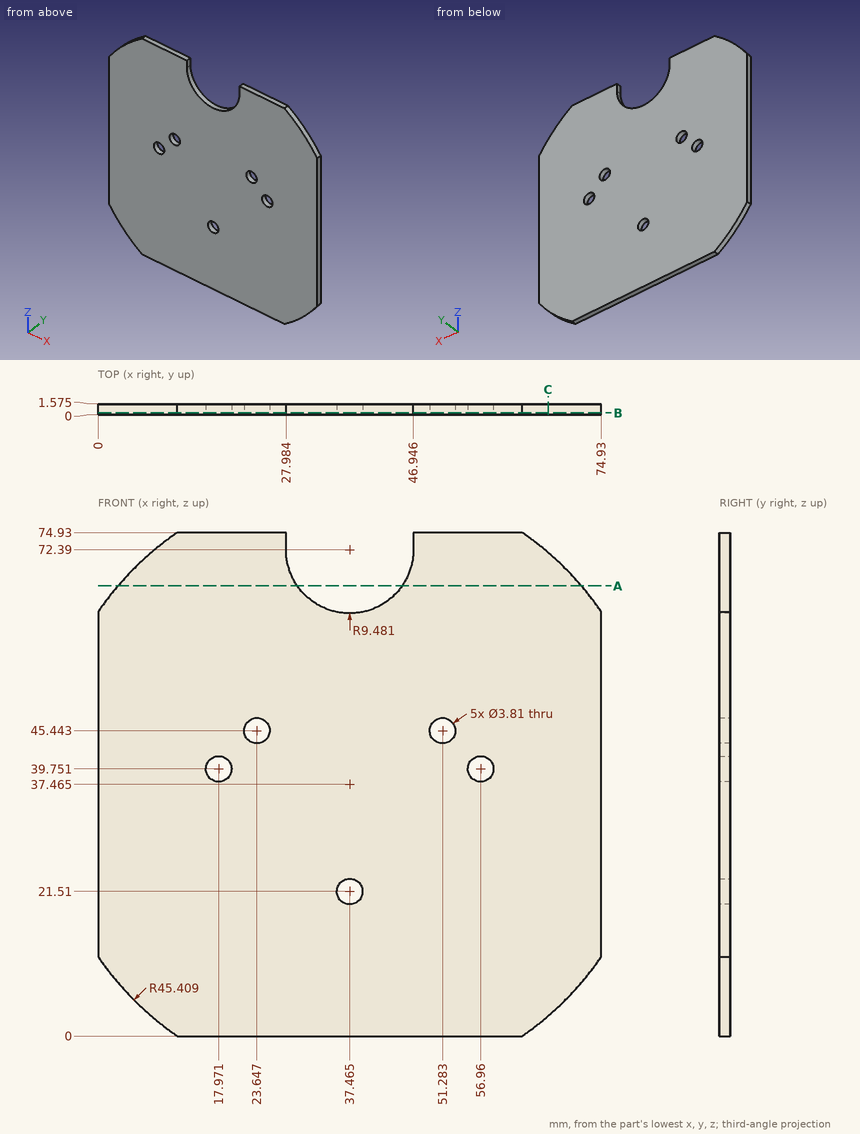
Here's the drawing with two shaded views (mm, measured from the low corner). I have some questions. Coordinates: 2 decimals unless noted, no trailing zeros. Write each loop counter-clockwise with the first axis right and the second up, starting at its lowest first coordinate (ties: lowest second). Pieces come first, ordered by that corner, then holes. Notation, with made-up numbers: (68, 71.5) - (108, 71.5) arc R29 ccw to (108, 96.5) - close; hole circle Ø8 at (21.5, -36). An arc over 180 degrees is marked (long way). Return JSON: item names as keys, results as strings.
Q1. Please list where these lines run through material, in increasing order: L1, parallel to X at y = 0.7, z = 41.5 (1 decimal); L2, parallel to Z at x = 56, y = 1.45 (1 decimal); L3, parallel to Z at x = 24, y = 0.8 (1 decimal). Write a range as from..to.
Computed values:
{"L1": "x = 0..17.2, 18.7..56.2, 57.7..74.9", "L2": "z = 0..38.1, 41.4..74.9", "L3": "z = 0..43.6, 47.3..74.9"}
Q2. I'm going to push a flat-ended pin straight in: pin 1 Ø2.5 at (x, z) = (23.65, 45.44) entering from -Y. Where does the tip first touch, or does it pass through?
Computed values:
{"pin 1": "passes through"}
Q3. If we section it at A-A (z = 67): Please give me the cut outline in (x, y) (1 decimal).
Computed values:
{"outline": "(3, 0) - (29.7, 0) - (29.7, 1.6) - (3, 1.6) - close; (45.3, 0) - (72, 0) - (72, 1.6) - (45.3, 1.6) - close"}
Q4. If we section it at B-B (y = 0.25): Count the separate pieces of the cut face and the enclosed holes in it, then the cut area to 3 significant figures.
Computed values:
{"separate pieces": "1", "enclosed holes": "5", "area": "5,120 mm2"}
Q5. If we section it at C-C (x = 67): Please give me the cut outline in (y, z) (1 decimal).
Computed values:
{"outline": "(0, 3) - (1.6, 3) - (1.6, 72) - (0, 72) - close"}
